Input: dimensioned drawing with shaded views. Units: mm. Origin: part minimum x, y, z. A direction names the side the tool comes from. Round coordinates to 2 decimals unless told otherwise and drop trailing zeros. Loops run counter-clockwise (first coordinate to the right, second up) from the corner with the lowest first, then second, coordinate; pieces in that order, holes last. Notation, with made-up numbers: M 71,-22 L 130,-22 A10 ccw 130,-9 Z; hole C 18,-32 d11. An arc over 180 degrees is marked long. Answer as CSV lines item,"result". Start each with the question number.
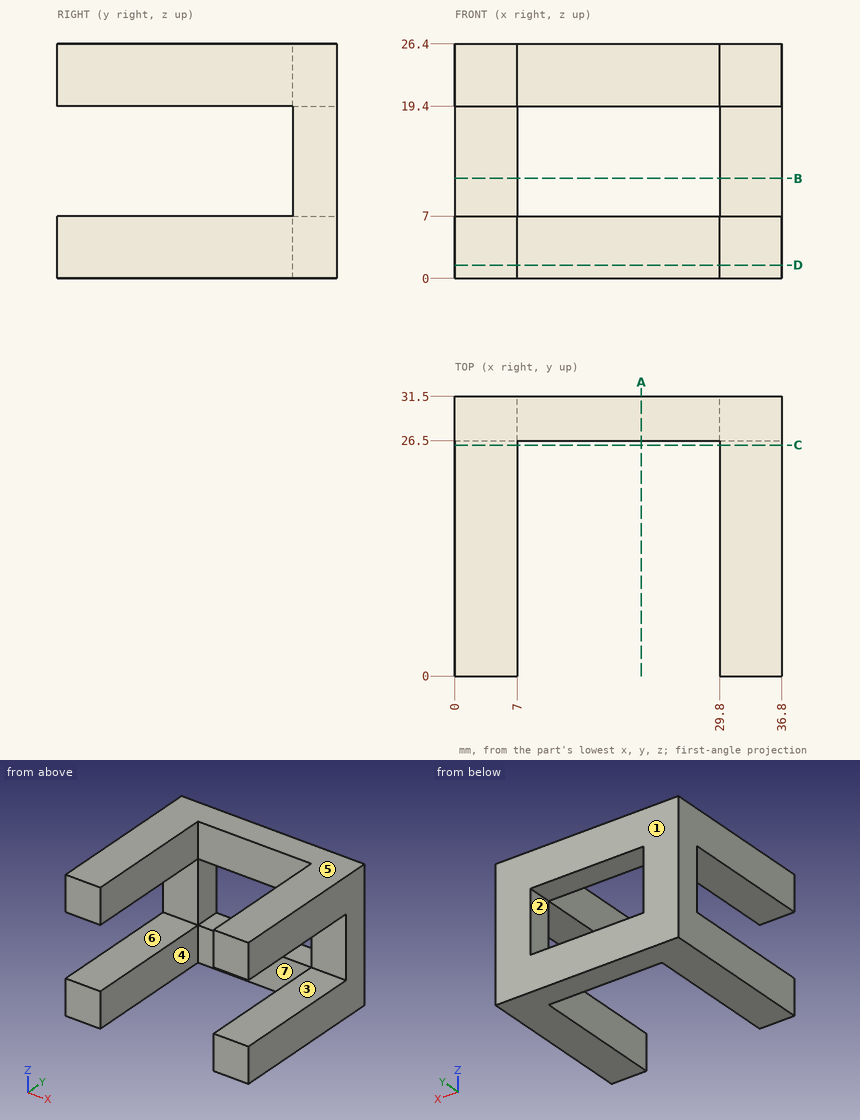
1) Contact query for flat-ended pins moving along their axis: pin 1 Ø6 at (x, y) = (25.5, 13) entering from -Z; pin 2 Ø5.5 at (x, z) = (14, 3) entering from -Y. Output: stop coordinate, or through.
2) Access query for the marked faces 1, 2, 3 and 4. Directions: +Z, -Z, +X, -X, +Y, -Y. A direction counts if a zero-diameter tool reaches every point of the face in a straight line with its end or side. Return the directions, or none.
3) Section A-A, the plane x = 21. Return loops of the section in (y, z), and give its area (3 significant figures).
4) Section C-C, the plane y = 26. Return loops of the section in (x, z), and give its area (3 significant figures).
5) Mould query, pull axis Z, two halves, no side actions, for the marked faces 5, 6 and 7. Classes: pulls with the +Z half, pulls with the -Z half, needs draft (parallel to the pull), parting line crosses it, or undercut.
6) Section B-B, the plane z = 11.25. Return loops of the section in (x, y).
7) Ray query, line 1 along X through (y, z) = (16.5, 25.25); line 2 along Z through (x, y) = (4, 16); line 3 along Y through (x, z) = (32, 10.5). Return the intervals inside material, ascending.
8) Section D-D, the plane z = 1.5. Return loops of the section in (x, y), and give its area (3 significant figures).
Findings below:
1,pin 1,"through"
1,pin 2,"y = 26.5"
2,face 1,"+Z, -Z, +X, -X, +Y"
2,face 2,"+Y, -Y"
2,face 3,"+X, -X, -Y"
2,face 4,"+Z, -Z, -Y"
3,outline,"M 26.5,0 L 31.5,0 L 31.5,7 L 26.5,7 Z; M 26.5,19.4 L 31.5,19.4 L 31.5,26.4 L 26.5,26.4 Z"
3,area,"70.0 mm²"
4,outline,"M 0,0 L 7,0 L 7,7 L 0,7 Z; M 0,19.4 L 7,19.4 L 7,26.4 L 0,26.4 Z; M 29.8,0 L 36.8,0 L 36.8,7 L 29.8,7 Z; M 29.8,19.4 L 36.8,19.4 L 36.8,26.4 L 29.8,26.4 Z"
4,area,"196 mm²"
5,face 5,"pulls with the +Z half"
5,face 6,"undercut"
5,face 7,"needs draft"
6,outline,"M 0,26.5 L 7,26.5 L 7,31.5 L 0,31.5 Z; M 29.8,26.5 L 36.8,26.5 L 36.8,31.5 L 29.8,31.5 Z"
7,line 1,"0 to 7, 29.8 to 36.8"
7,line 2,"0 to 7, 19.4 to 26.4"
7,line 3,"26.5 to 31.5"
8,outline,"M 0,0 L 7,0 L 7,26.5 L 29.8,26.5 L 29.8,0 L 36.8,0 L 36.8,31.5 L 0,31.5 Z"
8,area,"555 mm²"
